```python
from build123d import *

# Parameters (mm, degrees)
BOSS_EXTRUDE1_DEPTH = 1.524


with BuildPart() as part:
    # Sketch1 → Boss-Extrude1 (new body)
    with BuildSketch(Plane.XY):
        with BuildLine():
            Line((299.496674555, 247.083909986), (293.228442315, 248.191486466))
            Line((293.228442315, 248.191486466), (292.963264261, 246.690734455))
            Line((292.963264261, 246.690734455), (299.231496501, 245.583157975))
            ThreePointArc((299.231496501, 245.583157975), (301.853890913, 233.138709027), (311.755483248, 225.157497886))
            ThreePointArc((311.755483248, 225.157497886), (342.378628376, 201.501430101), (379.736207542, 191.411938565))
            ThreePointArc((379.736207542, 191.411938565), (367.282944414, 188.133579217), (354.433282196, 187.286476253))
            ThreePointArc((354.433282196, 187.286476253), (354.075780486, 186.801693195), (353.711488573, 186.321991739))
            Line((353.711488573, 186.321991739), (59.210439319, 228.618287464))
            ThreePointArc((59.210439319, 228.618287464), (46.845732275, 234.131121821), (34.989718338, 240.66658328))
            ThreePointArc((34.989718338, 240.66658328), (21.739819765, 249.170959745), (13.469532472, 262.568219888))
            ThreePointArc((13.469532472, 262.568219888), (14.473805053, 264.820038124), (16.64661192, 263.65463729))
            ThreePointArc((16.64661192, 263.65463729), (27.881645016, 252.981360845), (42.038095614, 246.677417222))
            ThreePointArc((42.038095614, 246.677417222), (47.204267049, 247.59528857), (51.319192238, 250.850930717))
            ThreePointArc((51.319192238, 250.850930717), (53.712623356, 252.761043669), (56.030286878, 254.76241315))
            Line((56.030286878, 254.76241315), (60.009228178, 249.866621656))
            Line((60.009228178, 249.866621656), (61.191894588, 250.827806426))
            Line((61.191894588, 250.827806426), (57.156306316, 255.793297808))
            ThreePointArc((57.156306316, 255.793297808), (63.269330312, 262.174956241), (68.631929607, 269.198997493))
            ThreePointArc((68.631929607, 269.198997493), (70.672937053, 278.271974974), (77.97930542, 284.025375103))
            ThreePointArc((77.97930542, 284.025375103), (75.025286429, 278.530980407), (75.355674106, 272.301578731))
            ThreePointArc((75.355674106, 272.301578731), (89.522712553, 279.763084543), (101.575381834, 290.304062227))
            ThreePointArc((101.575381834, 290.304062227), (105.298186283, 293.444448732), (109.921107262, 294.977387738))
            ThreePointArc((109.921107262, 294.977387738), (106.645115294, 290.563839268), (104.441699592, 285.528316185))
            ThreePointArc((104.441699592, 285.528316185), (105.901175076, 281.967449489), (109.74705726, 282.10540072))
            ThreePointArc((109.74705726, 282.10540072), (117.575446144, 283.528434685), (125.519570472, 283.081683228))
            ThreePointArc((125.519570472, 283.081683228), (131.283660572, 283.993726612), (135.76973662, 287.726243123))
            ThreePointArc((135.76973662, 287.726243123), (144.425837897, 293.107350234), (153.959513951, 296.711989461))
            ThreePointArc((153.959513951, 296.711989461), (159.650281584, 297.625042258), (165.406340408, 297.331293248))
            ThreePointArc((165.406340408, 297.331293248), (157.435124743, 294.404562686), (150.340503018, 289.738475081))
            ThreePointArc((150.340503018, 289.738475081), (167.005302639, 283.674185668), (184.616227681, 281.589366329))
            ThreePointArc((184.616227681, 281.589366329), (196.264753754, 282.403178747), (207.864638646, 283.742253372))
            Line((207.864638646, 283.742253372), (208.536964433, 277.452860551))
            Line((208.536964433, 277.452860551), (210.052330785, 277.614850731))
            Line((210.052330785, 277.614850731), (209.374499216, 283.955748378))
            ThreePointArc((209.374499216, 283.955748378), (227.881790203, 287.319954151), (246.095409129, 292.02120779))
            ThreePointArc((246.095409129, 292.02120779), (264.837645669, 295.417547796), (283.869742792, 294.652149172))
            ThreePointArc((283.869742792, 294.652149172), (300.377514826, 294.830345717), (316.730515739, 297.09256867))
            ThreePointArc((316.730515739, 297.09256867), (345.164765747, 299.513120241), (373.338877641, 304.050196657))
            ThreePointArc((373.338877641, 304.050196657), (393.078041438, 309.22946311), (413.38768552, 307.235034456))
            ThreePointArc((413.38768552, 307.235034456), (377.376618301, 298.266191923), (343.59946469, 282.892806069))
            ThreePointArc((343.59946469, 282.892806069), (321.044455039, 268.037495843), (300.562470929, 250.433603398))
            ThreePointArc((300.562470929, 250.433603398), (299.951704088, 248.78353273), (299.496674555, 247.083909986))
        make_face()
        with BuildLine():
            ThreePointArc((328.489226954, 199.182421434), (239.736316258, 213.199295119), (150.587010018, 224.42217807))
            ThreePointArc((150.587010018, 224.42217807), (145.688890945, 235.30713064), (142.759093928, 246.878217553))
            ThreePointArc((142.759093928, 246.878217553), (156.400368795, 248.593878404), (169.314596837, 243.8768257))
            ThreePointArc((169.314596837, 243.8768257), (196.80467914, 235.971060868), (225.395801684, 236.839078326))
            ThreePointArc((225.395801684, 236.839078326), (228.814239063, 235.855643459), (232.370913957, 235.909698546))
            ThreePointArc((232.370913957, 235.909698546), (247.490619756, 232.384573367), (260.020733604, 223.217880511))
            ThreePointArc((260.020733604, 223.217880511), (279.392290374, 215.299092788), (300.31360184, 215.812061861))
            ThreePointArc((300.31360184, 215.812061861), (313.259683309, 205.562804926), (328.489226954, 199.182421434))
        make_face(mode=Mode.SUBTRACT)
        with BuildLine():
            ThreePointArc((73.889360105, 231.521400998), (66.254747612, 236.297695357), (67.210403263, 245.252415788))
            ThreePointArc((67.210403263, 245.252415788), (70.194674676, 248.739861019), (73.390521828, 252.034509875))
            ThreePointArc((73.390521828, 252.034509875), (71.857270881, 241.734604422), (73.889360105, 231.521400998))
        make_face(mode=Mode.SUBTRACT)
        with BuildLine():
            ThreePointArc((113.10156747, 271.864588213), (123.557739252, 269.880401171), (134.129074941, 271.111412263))
            ThreePointArc((134.129074941, 271.111412263), (130.799977878, 248.854403449), (132.142963674, 226.389904395))
            ThreePointArc((132.142963674, 226.389904395), (114.719074022, 228.137810366), (97.284812247, 229.779036204))
            ThreePointArc((97.284812247, 229.779036204), (104.267717835, 248.98290031), (102.357800113, 269.327471609))
            ThreePointArc((102.357800113, 269.327471609), (107.682050527, 270.797739485), (113.10156747, 271.864588213))
        make_face(mode=Mode.SUBTRACT)
        with BuildLine():
            ThreePointArc((147.76400458, 278.362692247), (191.575815975, 273.02026788), (235.390344097, 278.340365744))
            ThreePointArc((235.390344097, 278.340365744), (257.681856345, 284.318322066), (280.730860591, 283.138964891))
            ThreePointArc((280.730860591, 283.138964891), (263.443829779, 271.830407732), (244.408703812, 263.806139622))
            ThreePointArc((244.408703812, 263.806139622), (218.447725967, 255.331740571), (194.986699965, 241.354327761))
            ThreePointArc((194.986699965, 241.354327761), (183.145599945, 244.034647083), (171.789821421, 248.329068519))
            ThreePointArc((171.789821421, 248.329068519), (157.383066968, 253.59262513), (142.123022895, 252.046450178))
            ThreePointArc((142.123022895, 252.046450178), (142.159172604, 263.976764596), (144.269250711, 275.719050545))
            ThreePointArc((144.269250711, 275.719050545), (146.057798086, 276.986446261), (147.76400458, 278.362692247))
        make_face(mode=Mode.SUBTRACT)
        with BuildLine():
            ThreePointArc((287.393755321, 282.043602932), (311.637801497, 288.812820245), (336.809005326, 288.893911982))
            ThreePointArc((336.809005326, 288.893911982), (307.570989951, 275.586964292), (284.906320156, 252.821878241))
            ThreePointArc((284.906320156, 252.821878241), (264.644027419, 253.656561884), (245.053092851, 248.417049837))
            ThreePointArc((245.053092851, 248.417049837), (224.280647922, 241.798667768), (202.516617159, 240.524142565))
            ThreePointArc((202.516617159, 240.524142565), (223.186364423, 251.866283632), (245.694745472, 258.884502671))
            ThreePointArc((245.694745472, 258.884502671), (267.708759315, 268.367301705), (287.393755321, 282.043602932))
        make_face(mode=Mode.SUBTRACT)
        with BuildLine():
            ThreePointArc((92.637447972, 265.466743872), (95.417062565, 247.800095776), (91.910427153, 230.263271083))
            ThreePointArc((91.910427153, 230.263271083), (86.111065378, 230.774336481), (80.310675632, 231.273599578))
            ThreePointArc((80.310675632, 231.273599578), (77.567314948, 243.850784297), (78.665529568, 256.676755136))
            ThreePointArc((78.665529568, 256.676755136), (85.404291465, 261.464676125), (92.637447972, 265.466743872))
        make_face(mode=Mode.SUBTRACT)
        with BuildLine():
            ThreePointArc((284.256505511, 247.772083796), (265.390502286, 248.627841972), (247.136907632, 243.783806264))
            ThreePointArc((247.136907632, 243.783806264), (242.957516866, 241.976149158), (238.694255905, 240.376293737))
            ThreePointArc((238.694255905, 240.376293737), (252.104272767, 235.759131886), (263.342997343, 227.108247207))
            ThreePointArc((263.342997343, 227.108247207), (279.254554924, 220.502299636), (296.480474873, 220.212662162))
            ThreePointArc((296.480474873, 220.212662162), (288.629921984, 233.221231814), (284.256505511, 247.772083796))
        make_face(mode=Mode.SUBTRACT)
    extrude(amount=BOSS_EXTRUDE1_DEPTH)


solid = part.part
```
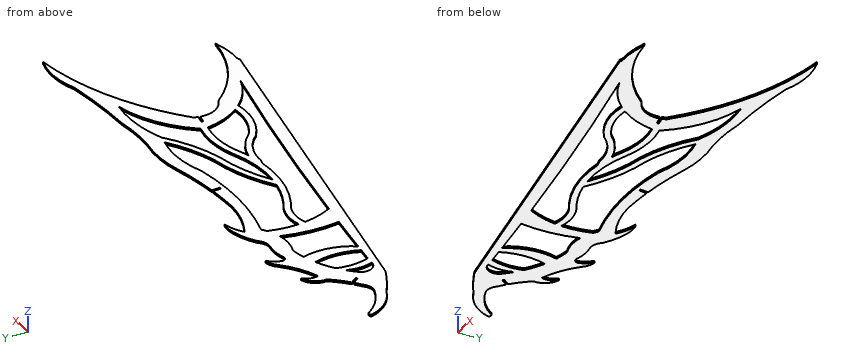
Verification items for the finished model (mm, model axes). Coordinates: 2 decimals unless noted, no trailing zeros. Write each loop counter-clockwise with the first axis right and the second up, starting at its lowest first coordinate (ties: lowest second). Pieces come first, ordered by that corner, then holes. Notation, with made-up numbers: M -30.75,16 L 1.25,16 A32 ccw 1.25,45 Z; hole C -19,3.5 d9. An arc over 180 degrees is marked long. One line per item, written item: value.
Item 1: Section check B-B, the plane z = 0.85. State how many separate pieces and enclosed holes the cut face has, plus the area to 3 significant figures.
Check sheet entries:
separate pieces: 1
enclosed holes: 7
area: 11,800 mm^2
Item 2: Section check A-A, the plane y = 210.5. Record the boundary of the cut face in (x, z), plus the area to 3 significant figures.
Check sheet entries:
outline: M 185.36,0 L 258.32,0 L 258.32,1.52 L 185.36,1.52 Z; M 306.12,0 L 327.64,0 L 327.64,1.52 L 306.12,1.52 Z
area: 144 mm^2
Item 3: Gauge pin test, flat ends, axial feed: pin 1 Ø12 at (x, y) = (366, 205) entering from -Z; pin 2 Ø12 at (x, y) = (181.5, 287) entering from +Z. Record the tip position at first contact, or that the pin passes through.
Check sheet entries:
pin 1: passes through
pin 2: stops at z = 1.52
Item 4: Scan lines: line 1 along Y through (x, z) = (265, 0.55); line 2 along Y through (x, z) = (331, 1.2); line 3 along Y through (x, z) = (166, 0.6). Record each from-to range of solid material in increasing order.
Check sheet entries:
line 1: y = 199.06 to 209.5, 220.25 to 226.07, 248.58 to 253.69, 266.91 to 272.67, 284.73 to 295.43
line 2: y = 189.58 to 208.13, 275.11 to 287.22, 289.48 to 298.04
line 3: y = 213.28 to 222.68, 245.78 to 251.35, 274.83 to 283.92
